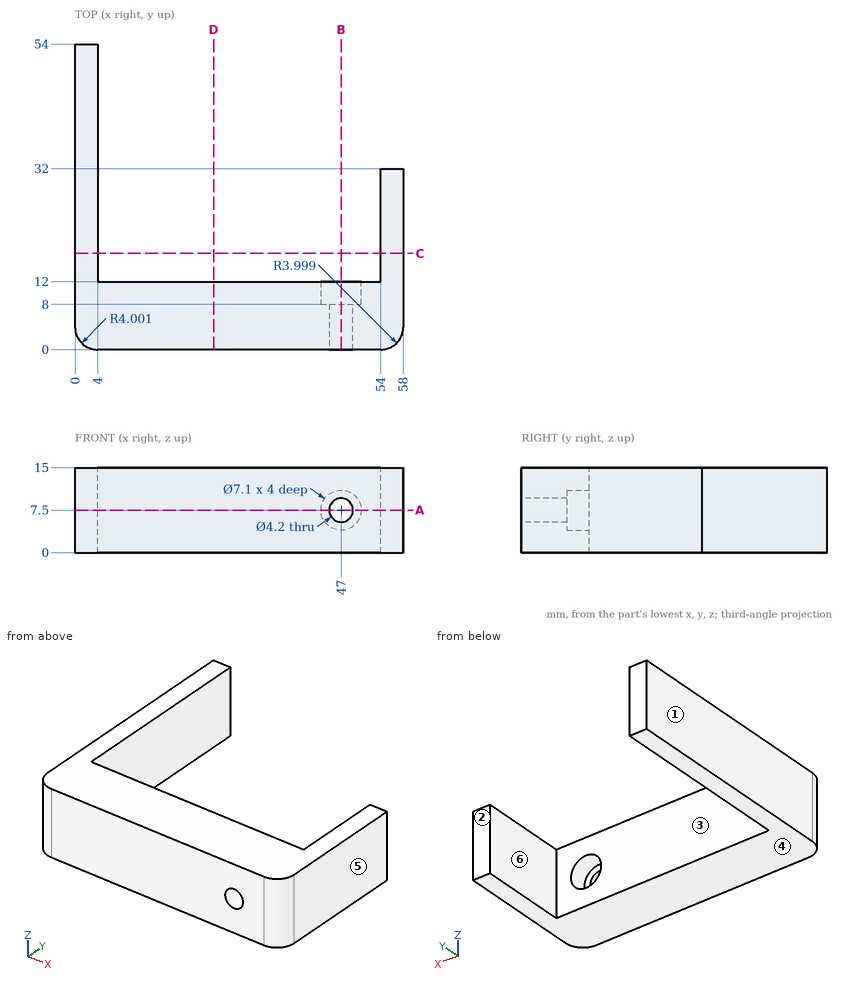
Check sheet for the drawn part. Datum: minimum x, y, z corner. Units: mm. A direction names the side the tool comes from. Give positions to 0.01 mm unless a question says otherwise; leave off trailing zeros. Write each loop counter-clockwise with the first axis right and the second up, starting at its lowest first coordinate (ties: lowest second). Pieces come first, ordered by that corner, then holes. Notation, with made-up numbers: M 12.5,9 L 70.5,9 A14 cw 70.5,14 Z; hole C 19,-36.5 d10. An arc over 180 degrees is marked long. One line per question, with ' | ' between items.
1) Thickness scan on line 1 along Z through (x, y) = (47, 9); line 2 along X through (y, z) = (27.5, 13.75); line 3 along Z through (x, y) = (47, 3.5). Record the ranges inside material, lowest first. Write a range as [from, to].
Result:
line 1: z = [0, 3.95], [11.05, 15] | line 2: x = [0, 4], [54, 58] | line 3: z = [0, 5.4], [9.6, 15]
2) Mould release check, pull along X, two halves, no side actions. Record for the marked faces 4, 5 and 6: released by +X, released by -X, zero draft, split by the parting line, or undercut.
Result:
face 4: zero draft | face 5: released by +X | face 6: undercut
3) Section check B-B on x = 47. Enter the section's corners in (y, z), plus the area to 3 significant figures.
Result:
outline: M 0,0 L 12,0 L 12,3.95 L 8,3.95 L 8,5.4 L 0,5.4 Z; M 0,9.6 L 8,9.6 L 8,11.05 L 12,11.05 L 12,15 L 0,15 Z | area: 118 mm2
4) Set-up check for the marked faces 1, 2 and 3: record each of +Z, -Z, +X, -X, +Y, -Y from which the full face is reachable in a straight line by a thin tool's end or side.
Result:
face 1: +Z, -Z, -X, +Y, -Y | face 2: +Z, -Z, +X, +Y | face 3: +Z, -Z, +Y
5) Section check D-D on x = 24.5. Enter the section's corners in (y, z).
Result:
outline: M 0,0 L 12,0 L 12,15 L 0,15 Z
6) Gauge pin test, flat ends, axial feed: pin 1 Ø1 at (x, z) = (37, 2.5) entering from +Y; pin 2 Ø2 at (x, z) = (47.5, 6) entering from +Y; pin 3 Ø4.5 at (x, z) = (56.5, 10) entering from +Y. Record the tip position at first contact, or that the pin passes through.
Result:
pin 1: stops at y = 12 | pin 2: stops at y = 8 | pin 3: stops at y = 32
7) Section check C-C on y = 17. Enter the section's corners in (x, z), plus the area to 3 significant figures.
Result:
outline: M 0,0 L 4,0 L 4,15 L 0,15 Z; M 54,0 L 58,0 L 58,15 L 54,15 Z | area: 120 mm2
8) Section check A-A on z = 7.5. Enter the section's corners in (x, y), plus the area to 3 significant figures.
Result:
outline: M 0,4 A4 ccw 4,0 L 44.9,0 L 44.9,8 L 43.45,8 L 43.45,12 L 4,12 L 4,54 L 0,54 Z; M 49.1,0 L 54,0 A4 ccw 58,4 L 58,32 L 54,32 L 54,12 L 50.55,12 L 50.55,8 L 49.1,8 Z | area: 875 mm2
